Work out the finished part from the listing and answer in its coordinate system (mm). A direction names the side the tool comes from. Round coordinates to 2 decimals unless told otherwise and drop trailing zeros. Order: outer loops, then holes, each group sorted by start corner. A loop starts at its lowest first (then second) coordinate and runs counter-clockwise, first axis right, second up. Notation, with made-up numbers: M 7.5,42.25 L 63.5,42.25 A30 cw 63.5,73.25 Z; hole C -36.5,30.25 d6. An arc over 180 degrees is marked long. Return JSON: item names as keys, results as strings.
from build123d import *

# Parameters (mm, degrees)
F0_W     = 274.682402
F0_H     = 96.840292
F1_DEPTH = 200
F2_T     = -5
F3_W     = 274.682402
F3_H     = 96.840292
F3_W_2   = 37.139356
F3_H_2   = 73.845126
F3_W_3   = 45.392542
F3_H_3   = 45.392544
F3_W_4   = 45.392528
F4_DEPTH = 5
F6_DEPTH = 205
F7_W     = 182
F7_H     = 62
F8_DEPTH = 8


with BuildPart() as f1:
    # F0 (on Front) → F1 (new body)
    with BuildSketch(Plane.XZ):
        Rectangle(F0_W, F0_H)
    extrude(amount=F1_DEPTH)

    # F2
    f2_openings = [f1.faces().sort_by_distance(p)[0] for p in [
        (0, -200, 0),
    ]]
    offset(amount=F2_T, openings=f2_openings)

    # F3 (on face) → F4 (join)
    with BuildSketch(Plane.XZ.offset(200)):
        Rectangle(F3_W, F3_H)
        with Locations((-103.137672, -6.497583)):
            Rectangle(F3_W_2, F3_H_2, mode=Mode.SUBTRACT)
        with Locations((-5.090558, -3.619425)):
            Rectangle(F3_W_3, F3_H_3, mode=Mode.SUBTRACT)
        with Locations((90.336949, -3.619425)):
            Rectangle(F3_W_4, F3_H_3, mode=Mode.SUBTRACT)
    extrude(amount=F4_DEPTH)

    # F5 (on face) → F6 (join)
    with BuildSketch(Plane(origin=(0, 0, 0), x_dir=(-1, 0, 0), z_dir=(0, 1, 0))):
        Polygon((0, 119.112626), (-137.341201, 48.420146), (137.341201, 48.420146), align=None)
    extrude(amount=-F6_DEPTH)

    # F7 (on face) → F8 (join)
    with BuildSketch(Plane(origin=(0, 0, -48.420146), x_dir=(1, 0, 0), z_dir=(0, 0, -1))):
        with Locations((46.341201, 236)):
            Rectangle(F7_W, F7_H)
    extrude(amount=-F8_DEPTH)


solid = f1.part
Item 1: Find section B-B (x = -49). Determine the outline of the cut face in (y, z).
Output:
{"outline": "M -205,-48.42 L 0,-48.42 L 0,93.89 L -205,93.89 Z; hole M -200,-43.42 L -5,-43.42 L -5,43.42 L -200,43.42 Z"}
Item 2: Consider line 1 along X through (y, z) = (-184.5, 35.5); line 2 along Y through (x, z) = (-69, -17.5); line 3 along Z through (x, y) = (115, -187). Determine where each line is inside the solid, lowest interval first. Write a range as [from, to].
Output:
{"line 1": "x = [-137.34, -132.34], [132.34, 137.34]", "line 2": "y = [-205, -200], [-5, 0]", "line 3": "z = [-48.42, -43.42], [43.42, 59.92]"}
Item 3: Find section D-D (y = -210). Determine the outline of the cut face in (x, z).
Output:
{"outline": "M -44.66,-48.42 L 137.34,-48.42 L 137.34,-40.42 L -44.66,-40.42 Z"}
Item 4: Which of the six approach directions +Z, -Z, +X, -X, +Y, -Y give full straight-line access (tool end or side, diameter ignored) to faces 1 (the flat face through (45, -236, -40.42)), 2 (the flat face through (-44.659, -236, -44)), 3 (the flat face through (-132.341, -101, -1))?
Output:
{"face 1": "+Z, +X, -X, -Y", "face 2": "+Z, -Z, -X, -Y", "face 3": "none"}
Item 5: The mould has two halves that part along Z. Classify faces 4 (the flat face through (132.341, -101, -1)), 5 (the flat face through (67.71, -101.06, 84.26)), 6 (the flat face through (-2, -135, -48.42)): pulls with the +Z half, pulls with the -Z half, needs draft (parallel to the pull), parting line crosses it, or undercut.
Output:
{"face 4": "undercut", "face 5": "pulls with the +Z half", "face 6": "pulls with the -Z half"}
Item 6: Each of these flat-tipped pins is pushed along its axis until it touches: pin 1 (10 mm diameter, centred on y = -61.5, z = 80.5, fed in from -X); pin 2 (2 mm diameter, centred on y = -135.5, z = 69, fed in from -X); pin 3 (4 mm diameter, centred on y = -105, z = 87, fed in from -X); pin 4 (12 mm diameter, centred on x = 81, z = 86, fed in from -Y). Where does it stop, or does it pass through?
Output:
{"pin 1": "stops at x = -84.73", "pin 2": "stops at x = -99.3", "pin 3": "stops at x = -66.27", "pin 4": "passes through"}
Item 7: Find section C-C (z = -35.5). Determine the outline of the cut face in (x, y), plus the area to 3 significant figures.
Output:
{"outline": "M -137.34,-205 L -121.71,-205 L -121.71,-200 L -132.34,-200 L -132.34,-5 L 132.34,-5 L 132.34,-200 L -84.57,-200 L -84.57,-205 L 137.34,-205 L 137.34,0 L -137.34,0 Z", "area": "4,510 mm^2"}
Item 8: Find section A-A (z = -6). Determine the outline of the cut face in (x, y), plus the area to 3 significant figures.
Output:
{"outline": "M -137.34,-205 L -121.71,-205 L -121.71,-200 L -132.34,-200 L -132.34,-5 L 132.34,-5 L 132.34,-200 L 113.03,-200 L 113.03,-205 L 137.34,-205 L 137.34,0 L -137.34,0 Z; M -84.57,-205 L -27.79,-205 L -27.79,-200 L -84.57,-200 Z; M 17.61,-205 L 67.64,-205 L 67.64,-200 L 17.61,-200 Z", "area": "4,060 mm^2"}
